```python
from build123d import *

# Parameters (mm, degrees)
SKETCH1_W           = 140
SKETCH1_H           = 160
BOSS_EXTRUDE2_DEPTH = 3.175
CUT_EXTRUDE1_REACH  = 156.451
SKETCH3_W           = 3.175
SKETCH3_H           = 20
SKETCH3_W_2         = 20
SKETCH3_H_2         = 3.175


with BuildPart() as part:
    # Sketch1 → Boss-Extrude2 (new body)
    with BuildSketch(Plane.XY):
        with Locations((-5.981871877, 54.431521206)):
            Rectangle(SKETCH1_W, SKETCH1_H)
    extrude(amount=BOSS_EXTRUDE2_DEPTH)

    # Sketch3 → Cut-Extrude1 (cut, up to next)
    with BuildSketch(Plane.XY.offset(3.175), mode=Mode.PRIVATE) as cut_extrude1_sk1:
        with Locations((-74.394371877, -6.318478794)):
            Rectangle(SKETCH3_W, SKETCH3_H)
    cut_extrude1_tool1 = extrude(cut_extrude1_sk1.sketch, amount=-CUT_EXTRUDE1_REACH, mode=Mode.PRIVATE) & part.part
    # Sketch3 → Cut-Extrude1 (cut, up to next)
    with BuildSketch(Plane.XY.offset(3.175), mode=Mode.PRIVATE) as cut_extrude1_sk2:
        with Locations((-74.394371877, 34.181521206)):
            Rectangle(SKETCH3_W, SKETCH3_H)
    cut_extrude1_tool2 = extrude(cut_extrude1_sk2.sketch, amount=-CUT_EXTRUDE1_REACH, mode=Mode.PRIVATE) & part.part
    # Sketch3 → Cut-Extrude1 (cut, up to next)
    with BuildSketch(Plane.XY.offset(3.175), mode=Mode.PRIVATE) as cut_extrude1_sk3:
        with Locations((-74.394371877, 74.681521206)):
            Rectangle(SKETCH3_W, SKETCH3_H)
    cut_extrude1_tool3 = extrude(cut_extrude1_sk3.sketch, amount=-CUT_EXTRUDE1_REACH, mode=Mode.PRIVATE) & part.part
    # Sketch3 → Cut-Extrude1 (cut, up to next)
    with BuildSketch(Plane.XY.offset(3.175), mode=Mode.PRIVATE) as cut_extrude1_sk4:
        with Locations((-74.394371877, 115.181521206)):
            Rectangle(SKETCH3_W, SKETCH3_H)
    cut_extrude1_tool4 = extrude(cut_extrude1_sk4.sketch, amount=-CUT_EXTRUDE1_REACH, mode=Mode.PRIVATE) & part.part
    # Sketch3 → Cut-Extrude1 (cut, up to next)
    with BuildSketch(Plane.XY.offset(3.175), mode=Mode.PRIVATE) as cut_extrude1_sk5:
        with Locations((-5.981871877, -23.980978794)):
            Rectangle(SKETCH3_W_2, SKETCH3_H_2)
    cut_extrude1_tool5 = extrude(cut_extrude1_sk5.sketch, amount=-CUT_EXTRUDE1_REACH, mode=Mode.PRIVATE) & part.part
    # Sketch3 → Cut-Extrude1 (cut, up to next)
    with BuildSketch(Plane.XY.offset(3.175), mode=Mode.PRIVATE) as cut_extrude1_sk6:
        with Locations((-46.481871877, -23.980978794)):
            Rectangle(SKETCH3_W_2, SKETCH3_H_2)
    cut_extrude1_tool6 = extrude(cut_extrude1_sk6.sketch, amount=-CUT_EXTRUDE1_REACH, mode=Mode.PRIVATE) & part.part
    # Sketch3 → Cut-Extrude1 (cut, up to next)
    with BuildSketch(Plane.XY.offset(3.175), mode=Mode.PRIVATE) as cut_extrude1_sk7:
        with Locations((34.518128123, -23.980978794)):
            Rectangle(SKETCH3_W_2, SKETCH3_H_2)
    cut_extrude1_tool7 = extrude(cut_extrude1_sk7.sketch, amount=-CUT_EXTRUDE1_REACH, mode=Mode.PRIVATE) & part.part
    # Sketch3 → Cut-Extrude1 (cut, up to next)
    with BuildSketch(Plane.XY.offset(3.175), mode=Mode.PRIVATE) as cut_extrude1_sk8:
        with Locations((-46.481871877, 132.844021206)):
            Rectangle(SKETCH3_W_2, SKETCH3_H_2)
    cut_extrude1_tool8 = extrude(cut_extrude1_sk8.sketch, amount=-CUT_EXTRUDE1_REACH, mode=Mode.PRIVATE) & part.part
    # Sketch3 → Cut-Extrude1 (cut, up to next)
    with BuildSketch(Plane.XY.offset(3.175), mode=Mode.PRIVATE) as cut_extrude1_sk9:
        with Locations((-5.981871877, 132.844021206)):
            Rectangle(SKETCH3_W_2, SKETCH3_H_2)
    cut_extrude1_tool9 = extrude(cut_extrude1_sk9.sketch, amount=-CUT_EXTRUDE1_REACH, mode=Mode.PRIVATE) & part.part
    # Sketch3 → Cut-Extrude1 (cut, up to next)
    with BuildSketch(Plane.XY.offset(3.175), mode=Mode.PRIVATE) as cut_extrude1_sk10:
        with Locations((34.518128123, 132.844021206)):
            Rectangle(SKETCH3_W_2, SKETCH3_H_2)
    cut_extrude1_tool10 = extrude(cut_extrude1_sk10.sketch, amount=-CUT_EXTRUDE1_REACH, mode=Mode.PRIVATE) & part.part
    # Sketch3 → Cut-Extrude1 (cut, up to next)
    with BuildSketch(Plane.XY.offset(3.175), mode=Mode.PRIVATE) as cut_extrude1_sk11:
        with Locations((62.430628123, 115.181521206)):
            Rectangle(SKETCH3_W, SKETCH3_H)
    cut_extrude1_tool11 = extrude(cut_extrude1_sk11.sketch, amount=-CUT_EXTRUDE1_REACH, mode=Mode.PRIVATE) & part.part
    # Sketch3 → Cut-Extrude1 (cut, up to next)
    with BuildSketch(Plane.XY.offset(3.175), mode=Mode.PRIVATE) as cut_extrude1_sk12:
        with Locations((62.430628123, 74.681521206)):
            Rectangle(SKETCH3_W, SKETCH3_H)
    cut_extrude1_tool12 = extrude(cut_extrude1_sk12.sketch, amount=-CUT_EXTRUDE1_REACH, mode=Mode.PRIVATE) & part.part
    # Sketch3 → Cut-Extrude1 (cut, up to next)
    with BuildSketch(Plane.XY.offset(3.175), mode=Mode.PRIVATE) as cut_extrude1_sk13:
        with Locations((62.430628123, 34.181521206)):
            Rectangle(SKETCH3_W, SKETCH3_H)
    cut_extrude1_tool13 = extrude(cut_extrude1_sk13.sketch, amount=-CUT_EXTRUDE1_REACH, mode=Mode.PRIVATE) & part.part
    # Sketch3 → Cut-Extrude1 (cut, up to next)
    with BuildSketch(Plane.XY.offset(3.175), mode=Mode.PRIVATE) as cut_extrude1_sk14:
        with Locations((62.430628123, -6.318478794)):
            Rectangle(SKETCH3_W, SKETCH3_H)
    cut_extrude1_tool14 = extrude(cut_extrude1_sk14.sketch, amount=-CUT_EXTRUDE1_REACH, mode=Mode.PRIVATE) & part.part
    add(cut_extrude1_tool1.solids().sort_by_distance((-74.394372, -6.318479, 3.175))[0], mode=Mode.SUBTRACT)
    add(cut_extrude1_tool2.solids().sort_by_distance((-74.394372, 34.181521, 3.175))[0], mode=Mode.SUBTRACT)
    add(cut_extrude1_tool3.solids().sort_by_distance((-74.394372, 74.681521, 3.175))[0], mode=Mode.SUBTRACT)
    add(cut_extrude1_tool4.solids().sort_by_distance((-74.394372, 115.181521, 3.175))[0], mode=Mode.SUBTRACT)
    add(cut_extrude1_tool5.solids().sort_by_distance((-5.981872, -23.980979, 3.175))[0], mode=Mode.SUBTRACT)
    add(cut_extrude1_tool6.solids().sort_by_distance((-46.481872, -23.980979, 3.175))[0], mode=Mode.SUBTRACT)
    add(cut_extrude1_tool7.solids().sort_by_distance((34.518128, -23.980979, 3.175))[0], mode=Mode.SUBTRACT)
    add(cut_extrude1_tool8.solids().sort_by_distance((-46.481872, 132.844021, 3.175))[0], mode=Mode.SUBTRACT)
    add(cut_extrude1_tool9.solids().sort_by_distance((-5.981872, 132.844021, 3.175))[0], mode=Mode.SUBTRACT)
    add(cut_extrude1_tool10.solids().sort_by_distance((34.518128, 132.844021, 3.175))[0], mode=Mode.SUBTRACT)
    add(cut_extrude1_tool11.solids().sort_by_distance((62.430628, 115.181521, 3.175))[0], mode=Mode.SUBTRACT)
    add(cut_extrude1_tool12.solids().sort_by_distance((62.430628, 74.681521, 3.175))[0], mode=Mode.SUBTRACT)
    add(cut_extrude1_tool13.solids().sort_by_distance((62.430628, 34.181521, 3.175))[0], mode=Mode.SUBTRACT)
    add(cut_extrude1_tool14.solids().sort_by_distance((62.430628, -6.318479, 3.175))[0], mode=Mode.SUBTRACT)


solid = part.part
```
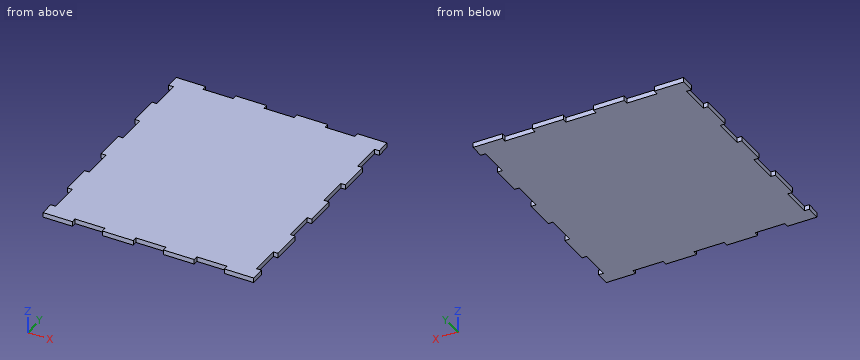
Source: CAD feature listing. Evaluate the final solid. Frame: model axes, mm. Round coordinates to 2 decimals unless told otherwise and drop trailing zeros. Write each loop counter-clockwise with the first axis right and the second up, starting at its lowest first coordinate (ties: lowest second). Pieces come first, ordered by that corner, then holes. Notation, with made-up numbers: M -20,45 L 1,45 A11 ccw 1,56 Z; hole C 65.5,62.5 d3. An arc over 180 degrees is marked long. Answer as a JSON object with one key per item and string values. Group by question number.
(1) Section query A-A on y = 30. Output: boundary loops of the cut face in (x, z) (3 decimals).
(2) First-contact query: pin 1 (1.6 mm diameter, centred on y = 74.5, z = 1, fed in from +X); pin 2 (1 mm diameter, centred on y = -1.5, z = 2, fed in from -X). Flat tips, straight axial feed; report the tip coordinate or a pass-through.
(3) Section query B-B on x = 35.5. Output: boundary loops of the cut face in (y, z) (3 decimals), then the cut area to 3 significant figures.
(4) Ray query, line 1 (X direction, y = -13, z = 0.3); line 2 (Y direction, x = 40, z = 0.7). Return the intervals inside material, ascending. Write a range as [from, to].
Computed values:
{
 "1": {"outline": "M -72.807,0 L 60.843,0 L 60.843,3.175 L -72.807,3.175 Z"},
 "2": {"pin 1": "x = 60.84", "pin 2": "x = -72.81"},
 "3": {"outline": "M -22.393,0 L 131.257,0 L 131.257,3.175 L -22.393,3.175 Z", "area": "488 mm^2"},
 "4": {"line 1": "[-72.81, 60.84]", "line 2": "[-22.39, 131.26]"}
}
